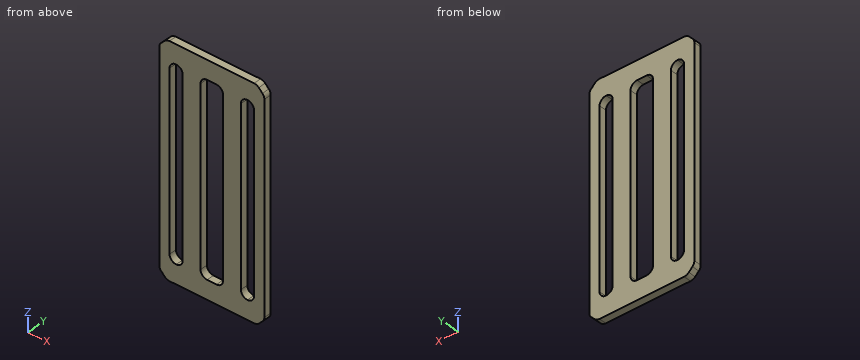
Autodesk Inventor part; units mm, degrees
ref_plane "YZ Plane" through (0, 0, 0) normal (1, 0, 0) x (0, 1, 0)
ref_plane "XZ Plane" through (0, 0, 0) normal (0, 1, 0) x (-1, 0, 0)
ref_plane "XY Plane" through (0, 0, 0) normal (0, 0, 1) x (1, 0, 0)
sketch "Szkic1" plane through (0, 0, 0) normal (0, 1, 0) x (-1, 0, 0)
  line L0 (14, 30) -> (-14, 30)
  line L1 (-14, 30) -> (-14, -30)
  line L2 (-14, -30) -> (14, -30)
  line L3 (14, -30) -> (14, 30)
  point P0 (0, 0)
  dimension "d0" = 28
  dimension "d1" = 14
  dimension "d2" = 60
  dimension "d3" = 30
extrude "Wyciągnięcie proste1" add sketch "Szkic1" along normal blind 2
sketch "Szkic2" plane through (0, 2, 0) normal (0, 1, 0) x (1, 0, 0)
  line L0 (-11.25, -25) -> (-7.75, -25)
  line L1 (-7.75, -25) -> (-7.75, 25)
  line L2 (-7.75, 25) -> (-11.25, 25)
  line L3 (-11.25, 25) -> (-11.25, -25)
  line L4 (7.75, -25) -> (11.25, -25)
  line L5 (11.25, -25) -> (11.25, 25)
  line L6 (11.25, 25) -> (7.75, 25)
  line L7 (7.75, 25) -> (7.75, -25)
  line L8 (-14, -30) -> (14, -30)
  line L9 (14, 30) -> (-14, 30)
  point P0 (0, 0)
  dimension "d6" = 3.5
  dimension "d7" = 3.5
  dimension "d8" = 5
  dimension "d9" = 0
  dimension "d10" = 5
  dimension "d11" = 0
  dimension "d12" = 15.5
  dimension "d13" = 7.75
extrude "Wyciągnięcie proste2" cut sketch "Szkic2" against normal blind 2
chamfer "Faza1" distance 2 angle 45 4 edges at (-14, 1, 30) (-14, 1, -30) (14, 1, -30) (14, 1, 30)
sketch "Szkic3" plane through (0, 2, 0) normal (0, 1, 0) x (1, 0, 0)
  line L0 (-3, -25) -> (3, -25)
  line L1 (3, -25) -> (3, 25)
  line L2 (3, 25) -> (-3, 25)
  line L3 (-3, 25) -> (-3, -25)
  point P0 (0, 0)
  dimension "d19" = 50
  dimension "d20" = 25
  dimension "d21" = 6
  dimension "d22" = 3
extrude "Wyciągnięcie proste3" cut sketch "Szkic3" against normal blind 2
fillet "Zaokrąglenie1" radius 1.75 12 edges at (3, 1, 25) (-7.75, 1, 25) (-11.25, 1, 25) (-3, 1, 25) (7.75, 1, 25) (-11.25, 1, -25) (-7.75, 1, -25) (-3, 1, -25) (3, 1, -25) (7.75, 1, -25) (11.25, 1, -25) (11.25, 1, 25)
fillet "Zaokrąglenie2" radius 1.75 8 edges at (-12, 1, -30) (-14, 1, -28) (12, 1, -30) (14, 1, -28) (12, 1, 30) (14, 1, 28) (-12, 1, 30) (-14, 1, 28)
properties part number "Holder"
Here's how the part is built. I have some questions about the finished solid (model axes, mm). Give positions to 0.01 mm unless a question says otherwise; leave off trailing zeros. Write each loop counter-clockwise with the first axis right and the second up, starting at its lowest first coordinate (ties: lowest second). Pieces come first, ordered by that corner, then holes. Notation, with made-up numbers: M 17.5,46 L 36.5,46 A21 ccw 36.5,69 Z; hole C 43,-38.75 d4. An arc over 180 degrees is marked long. Put each result on its own line as item: value. Start each with the question number.
Item 1: If we section it at A-A, the plane z = -15: Write out the boundary of the cut face in (x, y).
Item 2: If we section it at B-B, the plane x = -10.25: Write out the boundary of the cut face in (y, z), then the cut area to 3 significant figures.
Item 3: If we section it at C-C, the plane y = 1.4: Count the separate pieces of the cut face and the enclosed holes in it, then the cut area to 3 significant figures.
Item 4: I need wall thicknesses on L1, parallel to X at y = 0.25, z = 20; L2, parallel to Z at x = 1, y = 0.1; L3, parallel to Z at x = 8.75, y = 1.45. Which ranges of each line are inside material? Lowest first, please. Write a range as from..to.
Item 5: Will this pin go through, and if not, where does the flat tip stop? pin 1 (2 mm diameter, centred on x = -7.5, z = -15, fed in from -Y).
Values:
1. outline: M -14,0 L -11.25,0 L -11.25,2 L -14,2 Z; M -7.75,0 L -3,0 L -3,2 L -7.75,2 Z; M 3,0 L 7.75,0 L 7.75,2 L 3,2 Z; M 11.25,0 L 14,0 L 14,2 L 11.25,2 Z
2. outline: M 0,-30 L 2,-30 L 2,-24.83 L 0,-24.83 Z; M 0,24.83 L 2,24.83 L 2,30 L 0,30 Z
2. area: 20.7 mm²
3. separate pieces: 1
3. enclosed holes: 3
3. area: 1,030 mm²
4. L1: -14..-11.25, -7.75..-3, 3..7.75, 11.25..14
4. L2: -30..-25, 25..30
4. L3: -30..-24.83, 24.83..30
5. pin 1: y = 0
